Verification items for the finished model (mm, model axes). Round coordinates to 2 decimals unless told otherwise and drop trailing zeros. Answer as a JSON object with one key per item and string values. Group by question number.
(1) Sectioned sample at A-A on z = 5. Count the separate pieces of the cut face and the enclosed holes in it, and give its area (4 significant figures).
(2) Gauge pin test, flat ends, axial feed: pin 1 Ø3.5 at (x, y) = (-30.5, 86.5) entering from +Z; pin 2 Ø1 at (x, y) = (-11.5, 71.5) entering from +Z. Record the tip position at first contact, or that the pin passes through.
(3) Scan lines: L1, parallel to X at y = 42, z = 15.5; L2, parallel to X at y = -4, z = 13; L3, parallel to Z at x = -12.5, y = 25.5. Record each from-to range of solid material in increasing order. Write a range as from..to.
```python
from build123d import *

# Parameters (mm, degrees)
F0_W     = 85
F0_H     = 125
F1_DEPTH = 24
F2_W     = 57.5
F2_H     = 3
F3_DEPTH = 23
F4_R     = 2


# Not quite as in the source:
# - a feature names something its author has since deleted; it is built from what else it names


with BuildPart() as f1:
    # F0 (on Top) → F1 (new body)
    with BuildSketch(Plane.XY):
        with Locations((-7.3496025801, 34.134781265)):
            Rectangle(F0_W, F0_H)
    extrude(amount=F1_DEPTH)

    # F2 (on face) → F3 (cut)
    with BuildSketch(Plane.XY.offset(24)):
        with Locations((-16.0996025801, -18.365218735)):
            Rectangle(F2_W, F2_H)
        with Locations((-16.11783728, -3.365218735)):
            Rectangle(F2_W, F2_H)
        with Locations((-15.9132478945, 11.634781265)):
            Rectangle(F2_W, F2_H)
        with Locations((-16.0996025801, 26.634781265)):
            Rectangle(F2_W, F2_H)
        with Locations((-16.0996025801, 41.634781265)):
            Rectangle(F2_W, F2_H)
        with Locations((-16.0996025801, 56.634781265)):
            Rectangle(F2_W, F2_H)
        with Locations((-16.0996025801, 71.634781265)):
            Rectangle(F2_W, F2_H)
        with Locations((-16.0996025801, 86.634781265)):
            Rectangle(F2_W, F2_H)
    extrude(amount=-F3_DEPTH, mode=Mode.SUBTRACT)

    # F4
    f4_edges = [f1.edges().sort_by_distance(p)[0] for p in [
        (-16.099603, -19.865219, 24),
        (-16.099603, -16.865219, 24),
        (12.650397, -18.365219, 24),
        (-44.849603, -18.365219, 24),
        (-16.117837, -1.865219, 24),
        (-16.117837, -4.865219, 24),
        (-44.867837, -3.365219, 24),
        (12.632163, -3.365219, 24),
        (-49.849603, 34.134781, 24),
        (-7.349603, 96.634781, 24),
        (-7.349603, -28.365219, 24),
        (35.150397, 34.134781, 24),
        (12.650397, 26.634781, 24),
        (-16.099603, 28.134781, 24),
        (-44.849603, 26.634781, 24),
        (-16.099603, 25.134781, 24),
        (12.836752, 11.634781, 24),
        (-15.913248, 13.134781, 24),
        (-44.663248, 11.634781, 24),
        (-15.913248, 10.134781, 24),
        (-16.099603, 43.134781, 24),
        (-44.849603, 41.634781, 24),
        (-16.099603, 40.134781, 24),
        (12.650397, 41.634781, 24),
        (-16.099603, 58.134781, 24),
        (-44.849603, 56.634781, 24),
        (-16.099603, 55.134781, 24),
        (12.650397, 56.634781, 24),
        (-16.099603, 73.134781, 24),
        (-44.849603, 71.634781, 24),
        (-16.099603, 70.134781, 24),
        (12.650397, 71.634781, 24),
        (-16.099603, 88.134781, 24),
        (-44.849603, 86.634781, 24),
        (-16.099603, 85.134781, 24),
        (12.650397, 86.634781, 24),
    ]]
    fillet(f4_edges, radius=F4_R)


solid = f1.part
```
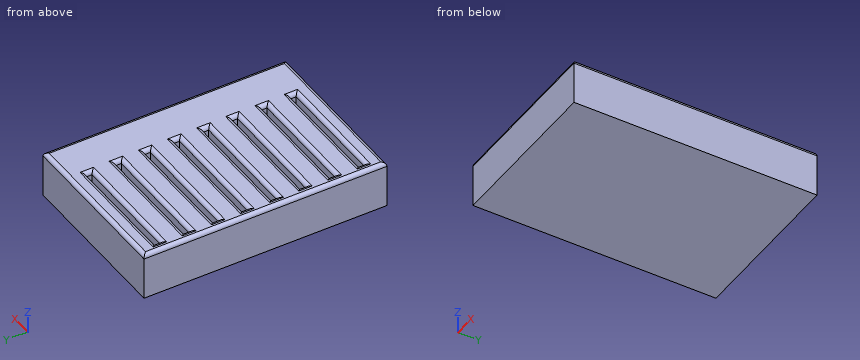
Computed values:
{
 "1": {"separate pieces": "1", "enclosed holes": "8", "area": "9,245 mm2"},
 "2": {"pin 1": "z = 23.18", "pin 2": "z = 1"},
 "3": {"L1": "-49.85..-44.85, 12.65..35.15", "L2": "-49.85..-44.87, 12.63..35.15", "L3": "0..1"}
}
